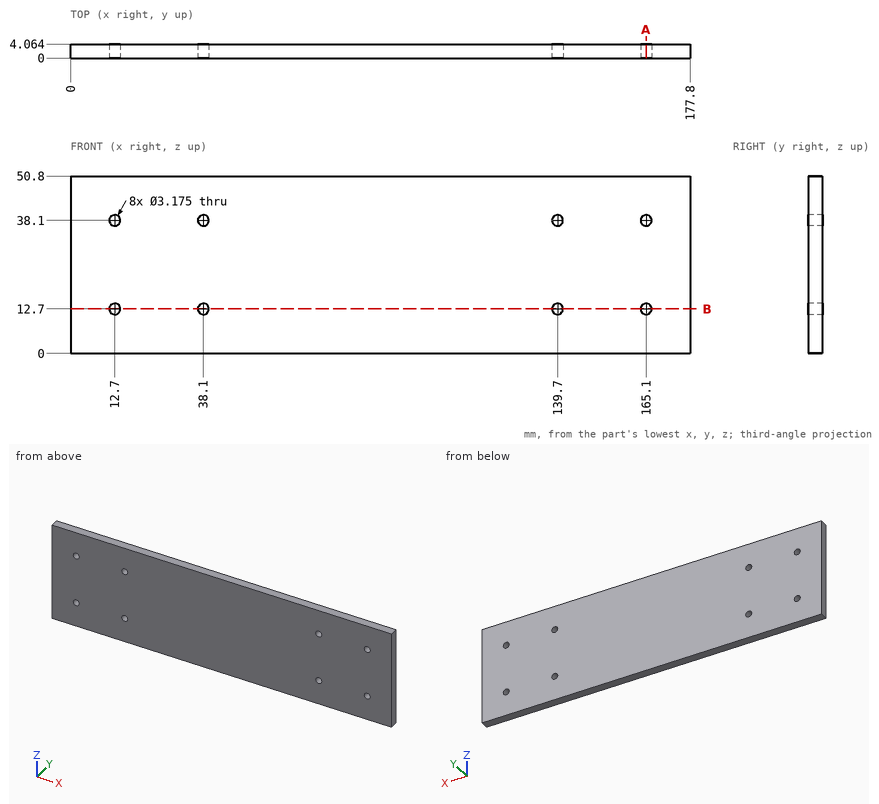
Here's the drawing with two shaded views (mm, measured from the low corner). I have some questions. Give positions to 0.01 mm unless a question says otherwise; leave off trailing zeros. Loops run counter-clockwise (first coordinate to the right, second up) from the corner with the lowest first, then second, coordinate; pieces in that order, holes last. Notation, with made-up numbers: M 46,86 L 58,86 A25 ccw 58,106 Z; hole C -3.75,54.5 d11. An arc over 180 degrees is marked long. Use one line per item in the form item = value. Start each with the question number.
Q1. I need wall thicknesses on line 1 along X through (y, z) = (3.6, 12.5); line 2 along Z through (x, y) = (38.1, 0.95). Which ranges of each line are inside material? Lowest first, please.
Q2. If we section it at A-A (x = 165.1): Write out the boundary of the cut face in (y, z).
Q3. If we section it at B-B (z = 12.7): Write out the boundary of the cut face in (x, y), then the cut area to 3 significant figures.
Q4. Will this pin go through, and if not, where does the flat tip stop? pin 1 Ø1.5 at (x, z) = (121.5, 8.5) entering from -Y.
Taken from the geometry:
q1.line_1 = 0 to 11.13, 14.27 to 36.53, 39.67 to 138.13, 141.27 to 163.53, 166.67 to 177.8
q1.line_2 = 0 to 11.11, 14.29 to 36.51, 39.69 to 50.8
q2.outline = M 0,0 L 4.06,0 L 4.06,11.11 L 0,11.11 Z; M 0,14.29 L 4.06,14.29 L 4.06,36.51 L 0,36.51 Z; M 0,39.69 L 4.06,39.69 L 4.06,50.8 L 0,50.8 Z
q3.outline = M 0,0 L 11.11,0 L 11.11,4.06 L 0,4.06 Z; M 14.29,0 L 36.51,0 L 36.51,4.06 L 14.29,4.06 Z; M 39.69,0 L 138.11,0 L 138.11,4.06 L 39.69,4.06 Z; M 141.29,0 L 163.51,0 L 163.51,4.06 L 141.29,4.06 Z; M 166.69,0 L 177.8,0 L 177.8,4.06 L 166.69,4.06 Z
q3.area = 671 mm^2
q4.pin_1 = 0
